Drawing for the job (mm, zero at the part's lowest x, y, z). Give positions to 0.01 mm unless a question says otherwise; leave off trailing zeros. Write each loop counter-clockwise with the first axis right and the second up, starting at its lowest first coordinate (ties: lowest second). Pieces come first, ordered by that corner, then holes.
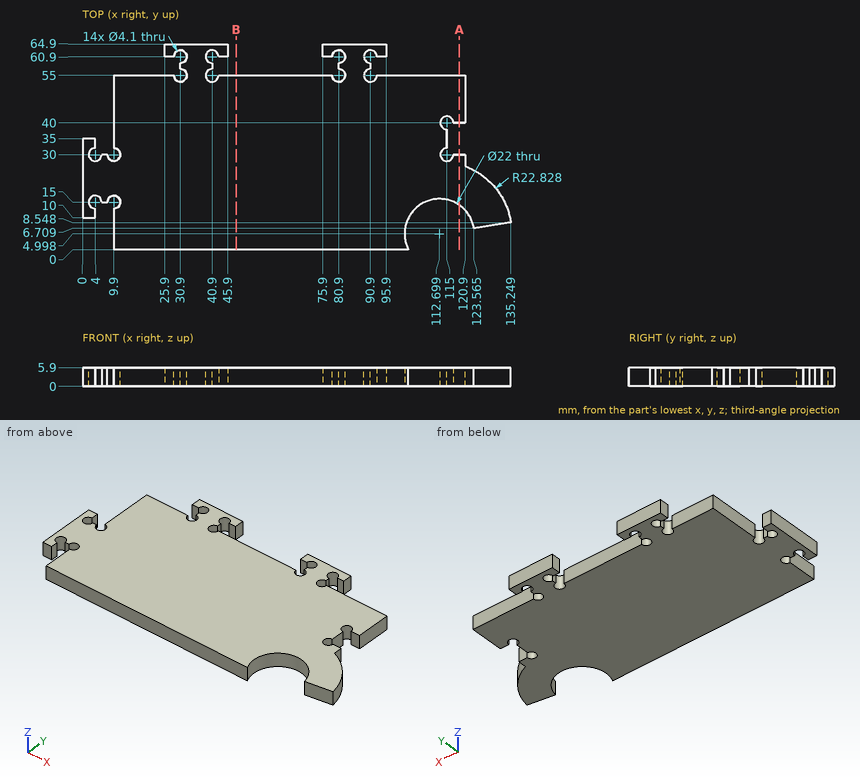
1. Slice it at B-B, the plane x = 48.5. Write the cut outline in (y, z).
Calculated:
outline: (0, 0) - (55, 0) - (55, 5.9) - (0, 5.9) - close
2. Probe probe 1 along X at (y, z) = (11, 0.65) (1 decimal); probe 2 along X at (y, z) = (29.5, 5.5); probe 3 along Y at (x, z) = (44, 2.8). List the from-to ranges inside material, lowest first.
Calculated:
probe 1: x = 0 to 4, 9.9 to 103.5, 121.9 to 134.7
probe 2: x = 0 to 2.01, 5.99 to 7.91, 11.89 to 113.01, 116.99 to 120.9
probe 3: y = 0 to 55, 60.9 to 64.9
3. Pin check, flat tips, straight feed: P1, Ø1.2, axis at x = 2.5, z = 1.5, coming from the +Y side; P2, Ø3.5, axis at x = 4, y = 30, coming from the -Z side (3 decimals); P3, Ø3, axis at y = 46, z = 3.5, coming from the +X side; P4, Ø0.5, axis at y = 57.5, z = 3.5, coming from the +X side. Stop position of each tip, or through.
Calculated:
P1: stops at y = 35
P2: passes through
P3: stops at x = 120.9
P4: stops at x = 90.9
4. Slice it at A-A, the plane x = 119. Write the cut outline in (y, z) (1 decimal), and give its area (3 significant figures).
Calculated:
outline: (14, 0) - (30, 0) - (30, 5.9) - (14, 5.9) - close; (40, 0) - (55, 0) - (55, 5.9) - (40, 5.9) - close
area: 183 mm2
